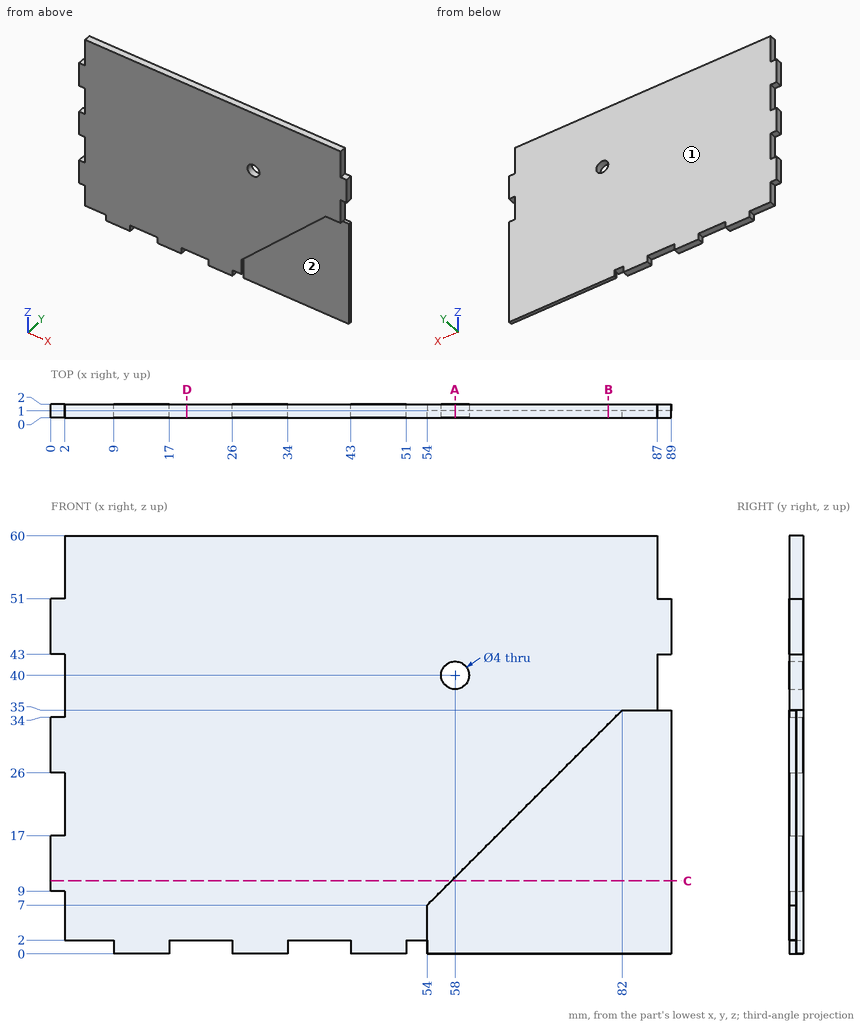
For this review, use the dimensioned drawing (mm, ordinates from the lowest corner) and the shaded views. A direction names the side the tool comes from. Give positions to 0.01 mm unless a question says otherwise; leave off trailing zeros. Write each loop counter-clockwise with the first axis right and the second up, starting at its lowest first coordinate (ties: lowest second). Pieces come first, ordered by that corner, then holes. Notation, with made-up numbers: M 52.5,-13.75 L 67.5,-13.75 A6 cw 67.5,-4.75 Z; hole C -32,34.5 d11. An arc over 180 degrees is marked long. Answer as a JSON object with one key per item and string values. Group by question number.
1) For line 1 along X through (y, z) = (0.95, 40); line 2 along Z through (x, y) = (58, 1.05); line 3 along Z through (x, y) = (18.5, 0.8), list the stretches that pass through material, from the lowest coordinate up.
2) We need section C-C (z = 10.5). Give the boundary of the cut face in (x, y), and give its area (4 significant figures).
3) We need section D-D (x = 19.5). Give the boundary of the cut face in (y, z), and give its area (3 significant figures).
4) We need section A-A (x = 58). Give the boundary of the cut face in (y, z).
5) Clearance check with flat-ended pins moving along their axes: pin 1 Ø0.5 at (y, z) = (0.5, 4.5) entering from +X; pin 2 Ø10 at (x, z) = (79.5, 13.5) entering from -Y; pin 3 Ø0.6 at (x, y) = (52.5, 1) entering from -Z. State where each tip first meets the part, or that it passes through.
6) Tool access review of the marked faces 1 and 2: name each direction out of +Z, -Z, +X, -X, +Y, -Y from which nothing blocks a thin tool from reaching the whole face with its end or side.
7) We need section B-B (x = 80). Give the boundary of the cut face in (y, z).
Answer key:
{
 "1": {"line 1": "x = 2 to 56, 60 to 87", "line 2": "z = 0 to 38, 42 to 60", "line 3": "z = 2 to 60"},
 "2": {"outline": "M 0,0 L 57.5,0 L 57.5,1 L 89,1 L 89,2 L 0,2 Z", "area": "146.5 mm²"},
 "3": {"outline": "M 0,2 L 2,2 L 2,60 L 0,60 Z", "area": "116 mm²"},
 "4": {"outline": "M 0,11 L 1,11 L 1,0 L 2,0 L 2,38 L 0,38 Z; M 0,42 L 2,42 L 2,60 L 0,60 Z"},
 "5": {"pin 1": "stops at x = 54", "pin 2": "stops at y = 1", "pin 3": "stops at z = 2"},
 "6": {"face 1": "+Z, -Z, +X, -X, +Y", "face 2": "-Z, +X, -Y"},
 "7": {"outline": "M 0,33 L 1,33 L 1,0 L 2,0 L 2,60 L 0,60 Z"}
}
